Autodesk Inventor part; units mm, degrees
ref_plane "YZ Plane" through (0, 0, 0) normal (1, 0, 0) x (0, 1, 0)
ref_plane "XZ Plane" through (0, 0, 0) normal (0, 1, 0) x (-1, 0, 0)
ref_plane "XY Plane" through (0, 0, 0) normal (0, 0, 1) x (1, 0, 0)
sketch "Sketch1" plane through (0, 0, 0) normal (0, 0, 1) x (1, 0, 0)
  line L0 (-3.175, 76.2) -> (3.175, 76.2)
  line L1 (3.175, 76.2) -> (3.175, -76.2)
  line L2 (3.175, -76.2) -> (-3.175, -76.2)
  line L3 (-3.175, -76.2) -> (-3.175, 76.2)
  line L4 (-3.175, 76.2) -> (3.175, -76.2) construction
  line L5 (3.175, 76.2) -> (-3.175, -76.2) construction
  point P0 (0, 0)
  dimension "d0" = 6.35
  dimension "d1" = 152.4
extrude "Extrusion1" add sketch "Sketch1" along normal mid plane 127
sketch "Sketch2" plane through (3.175, -76.2, 63.5) normal (1, 0, 0) x (0, 0, -1)
  line L0 (63.5, 83.6395) -> (81.4605, 101.6)
  line L1 (81.4605, 101.6) -> (63.5, 119.5605)
  line L2 (63.5, 119.5605) -> (45.5395, 101.6)
  line L3 (45.5395, 101.6) -> (63.5, 83.6395)
  line L4 (63.5, 83.6395) -> (63.5, 119.5605) construction
  line L5 (81.4605, 101.6) -> (45.5395, 101.6) construction
  line L6 (63.5, 83.6395) -> (88.9, 83.6395) construction
  line L7 (127, 152.4) -> (0, 152.4)
  point P0 (63.5, 76.2)
  point P1 (63.5, 101.6)
  point P2 (63.5, 152.4)
  point P3 (63.5, 101.6)
  dimension "d4" = 25.4
  dimension "d5" = 45
  dimension "d6" = 25.4
  dimension "d7" = 50.8
extrude "Extrusion2" cut sketch "Sketch2" against normal up to surface (6.35 mm away)
properties part number "x_axis_wood_mount" material "Wood (Birch)"
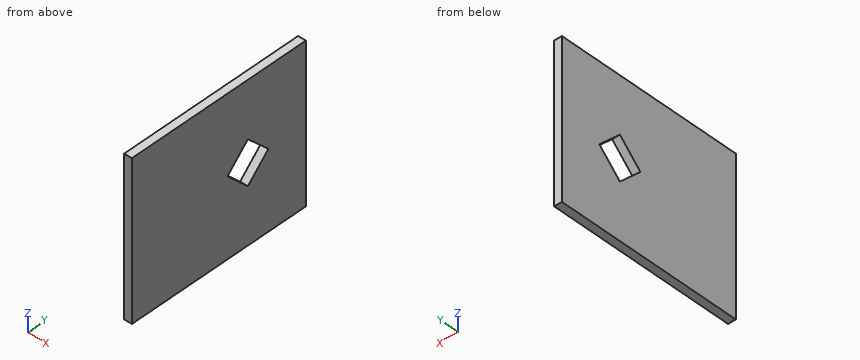
The model under review builds one solid part; all positions refer to its coordinate system, in mm. Coordinates: 2 decimals unless noted, no trailing zeros. Write each loop counter-clockwise with the first axis right and the second up, starting at its lowest first coordinate (ties: lowest second). Pieces come first, ordered by that corner, then holes. Notation, with made-up numbers: (22, 17) - (70, 17) arc R30 cw to (70, 52) - close; hole circle Ø11 at (-11.75, -36.5). An arc over 180 degrees is marked (long way). Answer in a Markdown table with one row per item. Add a question column.
Q1. Consider section C-C on z = -10. Give the boundary of the cut face in (x, y) (1 decimal).
Q2. To check wall thickness, follow line 1 along Y through (x, z) = (0.25, 6); line 2 along Y through (x, z) = (2.25, -11); line 3 along Z through (x, y) = (2, 28). State the ranges of each line that lie inside material, in increasing order. Write a range as from..to.
Q3. Consider section A-A on y = 12.5. Give the boundary of the cut face in (x, z) (1 decimal), then the cut area to 3 significant figures.
Q4. Consider section B-B on x = 0.5. Give the boundary of the cut face in (y, z), then the cut area to 3 significant figures.
Answers below:
| question | item | result |
|---|---|---|
| 1 | outline | (-3.2, -76.2) - (3.2, -76.2) - (3.2, 17.4) - (-3.2, 17.4) - close; (-3.2, 33.4) - (3.2, 33.4) - (3.2, 76.2) - (-3.2, 76.2) - close |
| 2 | line 1 | -76.2..13.44, 37.36..76.2 |
| 2 | line 2 | -76.2..18.44, 32.36..76.2 |
| 2 | line 3 | -63.5..-15.36, 15.36..63.5 |
| 3 | outline | (-3.2, -63.5) - (3.2, -63.5) - (3.2, -5.1) - (-3.2, -5.1) - close; (-3.2, 5.1) - (3.2, 5.1) - (3.2, 63.5) - (-3.2, 63.5) - close |
| 3 | area | 742 mm² |
| 4 | outline | (-76.2, -63.5) - (76.2, -63.5) - (76.2, 63.5) - (-76.2, 63.5) - close; hole (7.44, 0) - (25.4, -17.96) - (43.36, 0) - (25.4, 17.96) - close |
| 4 | area | 18,700 mm² |
